```python
from build123d import *

# Parameters (mm, degrees)
F0_R     = 2.25
F1_DEPTH = 24
F2_R     = 4
F2_R_2   = 2.25
F3_DEPTH = 10
F4_R     = 4


with BuildPart() as f1:
    # F0 (on Top) → F1 (new body)
    with BuildSketch(Plane.XY):
        Circle(F0_R)
    extrude(amount=F1_DEPTH)

    # F2 (on face) → F3 (join)
    with BuildSketch(Plane.XY.offset(24)):
        Circle(F2_R)
        Circle(F2_R_2, mode=Mode.SUBTRACT)
        Circle(F2_R_2)
    extrude(amount=F3_DEPTH)

    # F4
    f4_edges = [f1.edges().sort_by_distance(p)[0] for p in [
        (-4, 0, 34),
    ]]
    fillet(f4_edges, radius=F4_R)


solid = f1.part
```
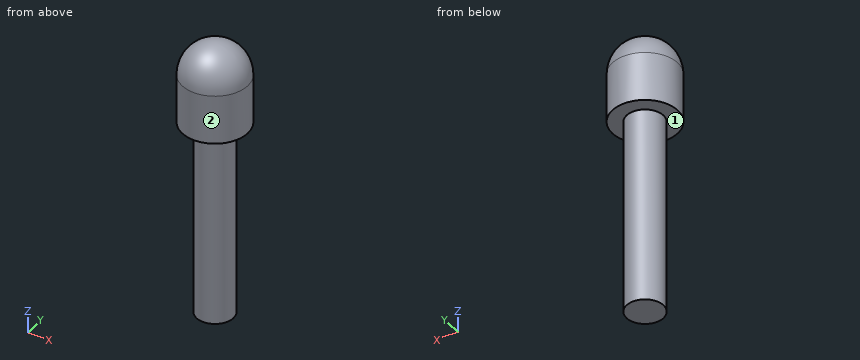
Input: part model. Units: mm. Frame: model coordinates. Face numbers are marked on the shaded views. A direction names the side the tool comes from. Give positions to 0.01 mm unless a question says otherwise; leave off trailing zeros. Order: outer loops, then holes, each group sorted by start corner. A loop starts at its lowest first (then second) coordinate and runs counter-clockwise, first axis right, second up. Notation, with made-up numbers: (81.25, 89) - (128.25, 89) arc R14 cw to (128.25, 104) - close; hole circle Ø11 at (35, 18). An arc over 180 degrees is marked (long way). One line per item, written item: value.
1. Reachability of the marked faces 1 and 2 from +Z, -Z, +X, -X, +Y, -Y: full face, straight path, thin tool, end or side. Return the list, or none.
Determined:
face 1: -Z
face 2: +Z, -Z
2. Cut plane A-A, the plane y = 0. Output: boundary loops of the cut face in (x, z), and give its area (3 significant figures).
Determined:
outline: (-4, 24) - (-2.25, 24) - (-2.25, 0) - (2.25, 0) - (2.25, 24) - (4, 24) - (4, 30) arc R4 ccw to (-4, 30) - close
area: 181 mm2
3. Line query: probe 1 along Y at (x, z) = (-1, 9.5); probe 2 along X at (y, z) = (-1, 27); probe 3 along X at (y, z) = (0.5, 21). Output: solid intervals per line, ascending.
Determined:
probe 1: -2.02 to 2.02
probe 2: -3.87 to 3.87
probe 3: -2.19 to 2.19
4. Pin query (flat end, axial travel): pin 1 Ø2 at (x, z) = (-1.5, 3.5) entering from +Y; pin 2 Ø1.5 at (x, z) = (-1.5, 15.5) entering from +Y. Return the tip coordinate at first contact, or that it passes through.
Determined:
pin 1: y = 2.19
pin 2: y = 2.12
5. Cut plane C-C, the plane z = 31.5. Output: boundary loops of the cut face in (x, y).
Determined:
outline: circle Ø7.42 at (0, 0)
6. Cut plane D-D, the plane z = 13. Output: boundary loops of the cut face in (x, y).
Determined:
outline: circle Ø4.5 at (0, 0)
